from build123d import *

# Parameters (mm, degrees)
SKETCH1_W                      = 30
SKETCH1_H                      = 50
BOSS_EXTRUDE1_DEPTH            = 4
F_3_0MM_DOWEL_HOLE1_AT_2_COUNT = 2
F_3_0MM_DOWEL_HOLE1_AT_2_PITCH = 11
F_3_0MM_DOWEL_HOLE1_AT_3_COUNT = 2
F_3_0MM_DOWEL_HOLE1_AT_3_PITCH = 21.09502311
F_3_0MM_DOWEL_HOLE1_AT_4_COUNT = 2
F_3_0MM_DOWEL_HOLE1_AT_4_PITCH = 18
M4_CLEARANCE_HOLE1_AT_2_COUNT  = 2
M4_CLEARANCE_HOLE1_AT_2_PITCH  = 20
FILLET1_R                      = 1
CHAMFER1_SIZE                  = 1


with BuildPart() as part:
    # Sketch1 → Boss-Extrude1 (new body)
    with BuildSketch(Plane.XY):
        with Locations((0, -14.5)):
            Rectangle(SKETCH1_W, SKETCH1_H)
    extrude(amount=BOSS_EXTRUDE1_DEPTH)

    # Sketch5 → 3.0mm Dowel Hole1 (revolve, cut)
    with BuildSketch(Plane(origin=(-9, 5.5, 4), x_dir=(0, -1, 0), z_dir=(1, 0, 0))):
        Polygon((0, 0), (0, 4), (1.75, 4), (1.5, 3.75), (1.5, 0.25), (1.75, 0), align=None)
    f_3_0mm_dowel_hole1 = revolve(axis=Axis((-9, 5.5, 10.35), (0, 0, -1)), mode=Mode.SUBTRACT)

    # 3.0mm Dowel Hole1 at 2: 3.0mm Dowel Hole1 ×2
    with Locations(*[(0, -i * F_3_0MM_DOWEL_HOLE1_AT_2_PITCH, 0) for i in range(1, F_3_0MM_DOWEL_HOLE1_AT_2_COUNT)]):
        add(f_3_0mm_dowel_hole1, mode=Mode.SUBTRACT)

    # 3.0mm Dowel Hole1 at 3: 3.0mm Dowel Hole1 ×2
    with Locations(*[Vector(0.853281834, -0.521450009, 0) * (i * F_3_0MM_DOWEL_HOLE1_AT_3_PITCH) for i in range(1, F_3_0MM_DOWEL_HOLE1_AT_3_COUNT)]):
        add(f_3_0mm_dowel_hole1, mode=Mode.SUBTRACT)

    # 3.0mm Dowel Hole1 at 4: 3.0mm Dowel Hole1 ×2
    with Locations(*[(i * F_3_0MM_DOWEL_HOLE1_AT_4_PITCH, 0, 0) for i in range(1, F_3_0MM_DOWEL_HOLE1_AT_4_COUNT)]):
        add(f_3_0mm_dowel_hole1, mode=Mode.SUBTRACT)

    # Sketch8 → M4 Clearance Hole1 (revolve, cut)
    with BuildSketch(Plane(origin=(-10, -34.5, 4), x_dir=(0, -1, 0), z_dir=(1, 0, 0))):
        Polygon((0, 0), (0, 4), (2.5, 4), (2.25, 3.75), (2.25, 0.25), (2.5, 0), align=None)
    m4_clearance_hole1 = revolve(axis=Axis((-10, -34.5, 10.35), (0, 0, -1)), mode=Mode.SUBTRACT)

    # M4 Clearance Hole1 at 2: M4 Clearance Hole1 ×2
    with Locations(*[(i * M4_CLEARANCE_HOLE1_AT_2_PITCH, 0, 0) for i in range(1, M4_CLEARANCE_HOLE1_AT_2_COUNT)]):
        add(m4_clearance_hole1, mode=Mode.SUBTRACT)

    # Fillet1
    fillet1_edges = [part.edges().sort_by_distance(p)[0] for p in [
        (15, -39.5, 2),
        (-15, -39.5, 2),
        (-15, 10.5, 2),
        (15, 10.5, 2),
    ]]
    fillet(fillet1_edges, radius=FILLET1_R)

    # Chamfer1
    chamfer1_edges = [part.edges().sort_by_distance(p)[0] for p in [
        (0, 10.5, 0),
        (0, 10.5, 4),
        (15, -14.5, 0),
        (0, -39.5, 0),
        (-15, -14.5, 0),
        (-14.707106781, 10.207106781, 0),
        (-14.707106781, -39.207106781, 0),
        (14.707106781, -39.207106781, 0),
        (14.707106781, 10.207106781, 0),
        (15, -14.5, 4),
        (-15, -14.5, 4),
        (0, -39.5, 4),
        (-14.707106781, 10.207106781, 4),
        (-14.707106781, -39.207106781, 4),
        (14.707106781, -39.207106781, 4),
        (14.707106781, 10.207106781, 4),
    ]]
    chamfer(chamfer1_edges, length=CHAMFER1_SIZE)


solid = part.part
Could you check a few things on this model? Use its own coordinates, in mm. Give positions to 0.01 mm unless a question says otherwise; leave off trailing zeros. Loops run counter-clockwise (first coordinate to the right, second up) from the corner with the lowest first, then second, coordinate; pieces in that order, holes last. Notation, with made-up numbers: (28.25, 37) -> (67.25, 37) arc R24 cw to (67.25, 76) -> close; hole circle Ø1 at (78, 18). An arc over 180 degrees is marked (long way). Answer as CSV lines item,"result". Start each with the question number.
(1) If we section it at B-B on z = 1.7: Write out the boundary of the cut face in (x, y), then the cut area to 3 significant figures.
(2) I'm going to push a flat-ended pin straight in: pin 1 Ø3.5 at (x, y) = (-10, -34.5) entering from -Z. Where does the tip first touch, or does it pass through?
(3) If we section it at C-C on y = -30: Write out the boundary of the cut face in (x, z).
(4) I need wall thicknesses on probe 1 along X at (y, z) = (-34.5, 1.9); probe 2 along X at (y, z) = (5.5, 2.4); probe 3 along Y at (x, z) = (9.5, 2.35). Which ranges of each line are inside material? Lowest first, please.
(5) If we section it at D-D on x = -9: Count the separate pieces of the cut face and the enclosed holes in it, then the cut area to 3 significant figures.
(6) We'd pull the mould along X, two halves only. Please class faces 1 (the cylindrical face through (-11.897, -35.71, 2.024)), 2 (the conical face through (14.355, 9.862, 0.507)), 3 (the conical face through (-14.362, 9.855, 3.493)), 4 (the flat face through (-0.2, 10, 3.5)): released by +X, released by -X, zero draft, split by the parting line, or undercut.
(7) If we section it at A-A on y = -5.5: Write out the boundary of the cut face in (x, z).
Computed:
1,outline,"(-15, -38.5) arc R1 ccw to (-14, -39.5) -> (14, -39.5) arc R1 ccw to (15, -38.5) -> (15, 9.5) arc R1 ccw to (14, 10.5) -> (-14, 10.5) arc R1 ccw to (-15, 9.5) -> close; hole circle Ø4.5 at (-10, -34.5); hole circle Ø3 at (-9, -5.5); hole circle Ø3 at (-9, 5.5); hole circle Ø3 at (9, -5.5); hole circle Ø3 at (9, 5.5); hole circle Ø4.5 at (10, -34.5)"
1,area,"1,440 mm2"
2,pin 1,"passes through"
3,outline,"(-15, 1) -> (-14, 0) -> (14, 0) -> (15, 1) -> (15, 3) -> (14, 4) -> (-14, 4) -> (-15, 3) -> close"
4,probe 1,"x = -15 to -12.25, -7.75 to 7.75, 12.25 to 15"
4,probe 2,"x = -15 to -10.5, -7.5 to 7.5, 10.5 to 15"
4,probe 3,"y = -39.5 to -36.69, -32.31 to -6.91, -4.09 to 4.09, 6.91 to 10.5"
5,separate pieces,"4"
5,enclosed holes,"0"
5,area,"157 mm2"
6,face 1,"undercut"
6,face 2,"released by +X"
6,face 3,"released by -X"
6,face 4,"zero draft"
7,outline,"(-15, 1) -> (-14, 0) -> (-10.75, 0) -> (-10.5, 0.25) -> (-10.5, 3.75) -> (-10.75, 4) -> (-14, 4) -> (-15, 3) -> close; (-7.5, 0.25) -> (-7.25, 0) -> (7.25, 0) -> (7.5, 0.25) -> (7.5, 3.75) -> (7.25, 4) -> (-7.25, 4) -> (-7.5, 3.75) -> close; (10.5, 0.25) -> (10.75, 0) -> (14, 0) -> (15, 1) -> (15, 3) -> (14, 4) -> (10.75, 4) -> (10.5, 3.75) -> close"
